from build123d import *

# Parameters (mm, degrees)
BOSS_EXTRUDE1_DEPTH = 6


with BuildPart() as part:
    # Sketch1 → Boss-Extrude1 (new body)
    with BuildSketch(Plane.XY):
        with BuildLine():
            Line((-53.972535853, 62.272181808), (-33.972535853, 62.272181808))
            Line((-33.972535853, 62.272181808), (-23.365934135, 51.66558009))
            Line((-23.365934135, 51.66558009), (-13.365934135, 51.66558009))
            Line((-13.365934135, 51.66558009), (4.134065865, 21.354690958))
            Line((4.134065865, 21.354690958), (4.134065865, 16.354690958))
            Line((4.134065865, 16.354690958), (0, 13.164382856))
            Line((0, 13.164382856), (0, 8.42299495))
            Line((0, 8.42299495), (4.271457393, 5.432088284))
            Line((4.271457393, 5.432088284), (-6.845344252, -27.755510623))
            Line((-6.845344252, -27.755510623), (-10.380878157, -31.291044529))
            Line((-10.380878157, -31.291044529), (-10.380878157, -36.291044529))
            Line((-10.380878157, -36.291044529), (-6.845344252, -39.826578434))
            Line((-6.845344252, -39.826578434), (-17.123685718, -80.844353089))
            ThreePointArc((-17.123685718, -80.844353089), (-19.962191865, -85.206806077), (-24.883760746, -86.899813152))
            Line((-24.883760746, -86.899813152), (-26.310778978, -86.899813152))
            ThreePointArc((-26.310778978, -86.899813152), (-33.291799073, -84.418493944), (-37.140699325, -78.087810456))
            Line((-37.140699325, -78.087810456), (-45.693891705, -36.899813152))
            Line((-45.693891705, -36.899813152), (-42.158357799, -33.364279246))
            Line((-42.158357799, -33.364279246), (-42.158357799, -28.364279246))
            Line((-42.158357799, -28.364279246), (-45.693891705, -24.828745341))
            Line((-45.693891705, -24.828745341), (-59.766941125, 1.66558009))
            Line((-59.766941125, 1.66558009), (-50.494368268, 1.66558009))
            ThreePointArc((-50.494368268, 1.66558009), (-46.444465696, 3.343104662), (-44.766941125, 7.393007234))
            Line((-44.766941125, 7.393007234), (-44.766941125, 21.96147854))
            Line((-44.766941125, 21.96147854), (-40.881118733, 25.10796616))
            Line((-40.881118733, 25.10796616), (-40.881118733, 31.10796616))
            Line((-40.881118733, 31.10796616), (-44.027606353, 34.993788551))
            Line((-44.027606353, 34.993788551), (-44.027606353, 40.822331304))
            ThreePointArc((-44.027606353, 40.822331304), (-47.203520392, 48.489666051), (-54.870855139, 51.66558009))
            Line((-54.870855139, 51.66558009), (-67.295502145, 51.66558009))
            Line((-67.295502145, 51.66558009), (-67.295502145, 57.971185507))
            Line((-67.295502145, 57.971185507), (-53.972535853, 62.272181808))
        make_face()
    extrude(amount=BOSS_EXTRUDE1_DEPTH)


solid = part.part
Design review of the part built by this model. Coordinates are the model's own, in mm. A direction names the side the tool comes from. Round coordinates to 2 decimals unless told otherwise and drop trailing zeros. Loops run counter-clockwise (first coordinate to the right, second up) from the corner with the lowest first, then second, coordinate; pieces in that order, holes last. Notation, with made-up numbers: (66, -8.75) - (121, -8.75) arc R17 cw to (121, 21.25) - close; hole circle Ø10 at (53.25, 80.25). An arc over 180 degrees is marked (long way). One line per item, written item: value. Start each with the question number.
1) Consider section C-C on y = 10. Give the boundary of the cut face in (x, z), then the cut area to 3 significant figures.
2) Consider section B-B on x = -57.5. Give the boundary of the cut face in (y, z), then the cut area to 3 significant figures.
3) Consider section D-D on x = -2.5. Give the boundary of the cut face in (y, z).
4) For faces 1 (the flat face through (4.134, 19, 3)), 2 (the flat face through (-55, 1.666, 3)), 3 (the flat face through (-60.7, 60.1, 3)), 4 (the flat face through (-8.64, -38.03, 2.96)), list the 3-axis set-ups (+Z, -Z, +X, -X, +Y, -Y) from which the entire face can be reached by the end or side of a thin tool; tool diameter is ignored.
5) Insertion check: pin 1 Ø1.8 at (x, z) = (-61, 3.5) entering from -Y; pin 2 Ø3 at (x, z) = (-17, 2) entering from +Y; pin 3 Ø1.5 at (x, z) = (-5, 1.5) entering from +Y. Each pin has a flat end and moves straight along its axis. Give the tip position at first contact, or say it passes through.
6) To check wall thickness, follow L1, parallel to X at y = 18, z = 3; L2, parallel to X at y = 10, z = 0.5; L3, parallel to Y at x = -52, z = 1.6. State the ranges of each line that lie inside material, in increasing order. Write a range as from..to.
7) Draft analysis for pull direction Y (two halves, no side actions). For faces 5 (the flat face through (-8.59, -29.5, 2.96)), 6 (the flat face through (-41.357, -57.782, 2.958)), 7 (the flat face through (-23, -11, 6)), state which applies: +Y half, -Y half, draft (parallel to the pull), parting line (faces both ways), or undercut.
Reported:
1. outline: (-44.77, 0) - (0, 0) - (0, 6) - (-44.77, 6) - close
1. area: 269 mm^2
2. outline: (-2.6, 0) - (1.67, 0) - (1.67, 6) - (-2.6, 6) - close; (51.67, 0) - (61.13, 0) - (61.13, 6) - (51.67, 6) - close
2. area: 82.4 mm^2
3. outline: (-14.78, 0) - (32.85, 0) - (32.85, 6) - (-14.78, 6) - close
4. face 1: +Z, -Z, +X, +Y
4. face 2: +Z, -Z, -X
4. face 3: +Z, -Z, -X, +Y
4. face 4: +Z, -Z, +X
5. pin 1: stops at y = 51.67
5. pin 2: stops at y = 51.67
5. pin 3: stops at y = 38.47
6. L1: x = -44.77..4.13
6. L2: x = -44.77..0
6. L3: y = -12.96..1.67, 51.28..62.27
7. face 5: undercut
7. face 6: -Y half
7. face 7: draft
